from build123d import *

# Parameters (mm, degrees)
PAD_DEPTH    = 1
PAD001_DEPTH = 3
PAD001_TAPER = 7
POCKET_DEPTH = 2.001
FILLET002_R  = 0.5


with BuildPart() as part:
    # Sketch005 → Pad (new body)
    with BuildSketch(Plane.XY):
        with BuildLine():
            Line((-35.5, 40.5), (35.5, 40.5))
            ThreePointArc((40.5, 35.5), (39.035534, 39.035534), (35.5, 40.5))
            Line((40.5, 35.5), (40.5, -35.5))
            ThreePointArc((35.5, -40.5), (39.035534, -39.035534), (40.5, -35.5))
            Line((35.5, -40.5), (-35.5, -40.5))
            ThreePointArc((-40.5, -35.5), (-39.035534, -39.035534), (-35.5, -40.5))
            Line((-40.5, -35.5), (-40.5, 35.5))
            ThreePointArc((-35.5, 40.5), (-39.035534, 39.035534), (-40.5, 35.5))
        make_face()
    extrude(amount=PAD_DEPTH)

    # Sketch004 → Pad001 (join)
    with BuildSketch(Plane.XY):
        with BuildLine():
            Line((-34.45, 39.45), (34.45, 39.45))
            ThreePointArc((39.45, 34.45), (37.985534, 37.985534), (34.45, 39.45))
            Line((39.45, 34.45), (39.45, -34.45))
            ThreePointArc((34.45, -39.45), (37.985534, -37.985534), (39.45, -34.45))
            Line((34.45, -39.45), (-34.45, -39.45))
            ThreePointArc((-39.45, -34.45), (-37.985534, -37.985534), (-34.45, -39.45))
            Line((-39.45, -34.45), (-39.45, 34.45))
            ThreePointArc((-34.45, 39.45), (-37.985534, 37.985534), (-39.45, 34.45))
        make_face()
    extrude(amount=-PAD001_DEPTH, taper=PAD001_TAPER)

    # Sketch006 → Pocket (cut, through all)
    with BuildSketch(Plane.XY.offset(-1)):
        with BuildLine():
            Line((-31, 36), (31, 36))
            ThreePointArc((36, 31), (34.535534, 34.535534), (31, 36))
            Line((36, 31), (36, -31))
            ThreePointArc((31, -36), (34.535534, -34.535534), (36, -31))
            Line((31, -36), (-31, -36))
            ThreePointArc((-36, -31), (-34.535534, -34.535534), (-31, -36))
            Line((-36, -31), (-36, 31))
            ThreePointArc((-31, 36), (-34.535534, 34.535534), (-36, 31))
        make_face()
    extrude(amount=POCKET_DEPTH, mode=Mode.SUBTRACT)

    # Fillet002
    fillet002_edges = [part.edges().sort_by_distance(p)[0] for p in [
        (0, 36, 1),
        (-34.535534, 34.535534, 1),
        (-36, 0, 1),
        (-34.535534, -34.535534, 1),
        (0, -36, 1),
        (34.535534, -34.535534, 1),
        (36, 0, 1),
        (34.535534, 34.535534, 1),
        (0, 40.5, 1),
        (-39.035534, 39.035534, 1),
        (-40.5, 0, 1),
        (-39.035534, -39.035534, 1),
        (0, -40.5, 1),
        (39.035534, -39.035534, 1),
        (40.5, 0, 1),
        (39.035534, 39.035534, 1),
    ]]
    fillet(fillet002_edges, radius=FILLET002_R)


solid = part.part
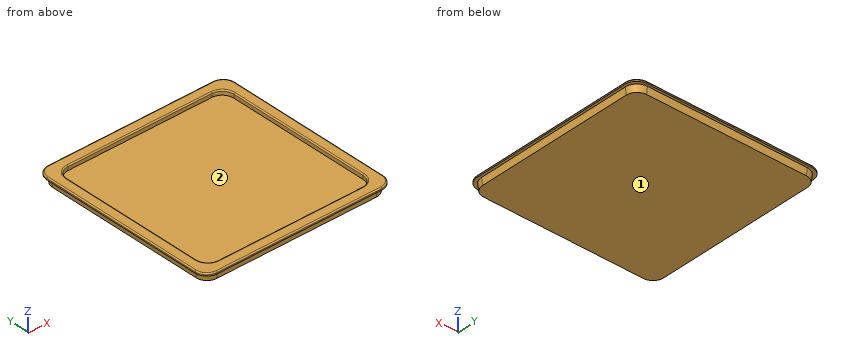
The listing builds one solid part. Answer for the finished solid, in the listing's coordinates (mm). Face numbers are marked on the shaded views. Round coordinates to 2 decimals unless told otherwise and drop trailing zeros. Answer in a Markdown table with one row per item. Add a question column.
1) Consider line 1 along Z through (x, y) = (7, -25); line 2 along X through (y, z) = (5.5, -0.1); line 3 along X through (y, z) = (-25, -0.9). Determine where each line is inside the solid, lowest interval first. Write a range as from..to.
2) Determine the mould class of the marked faces 1 and 2 for opening direction Y: pulls with the +Y half, pulls with the -Y half, needs draft (parallel to the pull), parting line crosses it, or undercut.
3) Flat-ended cylindrical pins translate along their axes: pin 1 Ø3 at (x, y) = (-25.5, -31) entering from +Z; pin 2 Ø2 at (y, z) = (-24.5, -2) entering from -X; pin 3 Ø0.8 at (y, z) = (-7.5, -0.5) entering from -X. Find the tip coordinate at first contact, or state that the pin passes through.
Findings below:
| question | item | result |
|---|---|---|
| 1 | line 1 | z = -3..-1 |
| 1 | line 2 | x = -39.44..-36, 36..39.44 |
| 1 | line 3 | x = -39.34..-36, 36..39.34 |
| 2 | face 1 | needs draft |
| 2 | face 2 | undercut |
| 3 | pin 1 | stops at z = -1 |
| 3 | pin 2 | stops at x = -39.33 |
| 3 | pin 3 | stops at x = -39.44 |
